For this review, use the dimensioned drawing (mm, ordinates from the lowest corner) and the shaded views. A direction names the side the tool comes from. Coordinates: 2 decimals unless noted, no trailing zeros. Loops run counter-clockwise (first coordinate to the right, second up) from the corner with the lowest first, then second, coordinate; pieces in that order, holes last. Notation, with made-up numbers: M -40,61.25 L -6,61.25 A30 ccw -6,98.25 Z; hole C -7.5,83 d2. An arc over 180 degrees is marked long. Write item = value, one per line. Start each with the question number.
Q1. We need section D-D on x = 15. Give the boundary of the cut face in (y, z), and give its area (3 significant figures).
Q2. For the marked faces 1 and 2, list the 3-axis set-ups (+Z, -Z, +X, -X, +Y, -Y) from which the entire face can be reached by the end or side of a thin tool; tool diameter is ignored.
Q3. Clearance check with flat-ended pins moving along their axes: pin 1 Ø1.5 at (x, z) = (12, 17) entering from +Y; pin 2 Ø10 at (x, y) = (14.5, 12.5) entering from +Z. State where each tip first meets the part, or that it passes through.
Q4. We need section B-B on x = 9. Give the boundary of the cut face in (y, z).
Q5. Mouldability with a two-part tool opening along Y and no side actions: class the marked faces 3, 4 and 5 as released by +Y, released by -Y, zero draft, split by the parting line, or undercut.
Q6. We need section A-A on z = 10. Give the boundary of the cut face in (x, y), and give its area (3 significant figures).
Q7. Wall thickness on probe 1 along X at (y, z) = (1.15, 10); probe 2 along Y at (x, z) = (9, 2.05): over which ranges is each line inside the solid? List them lowest first.
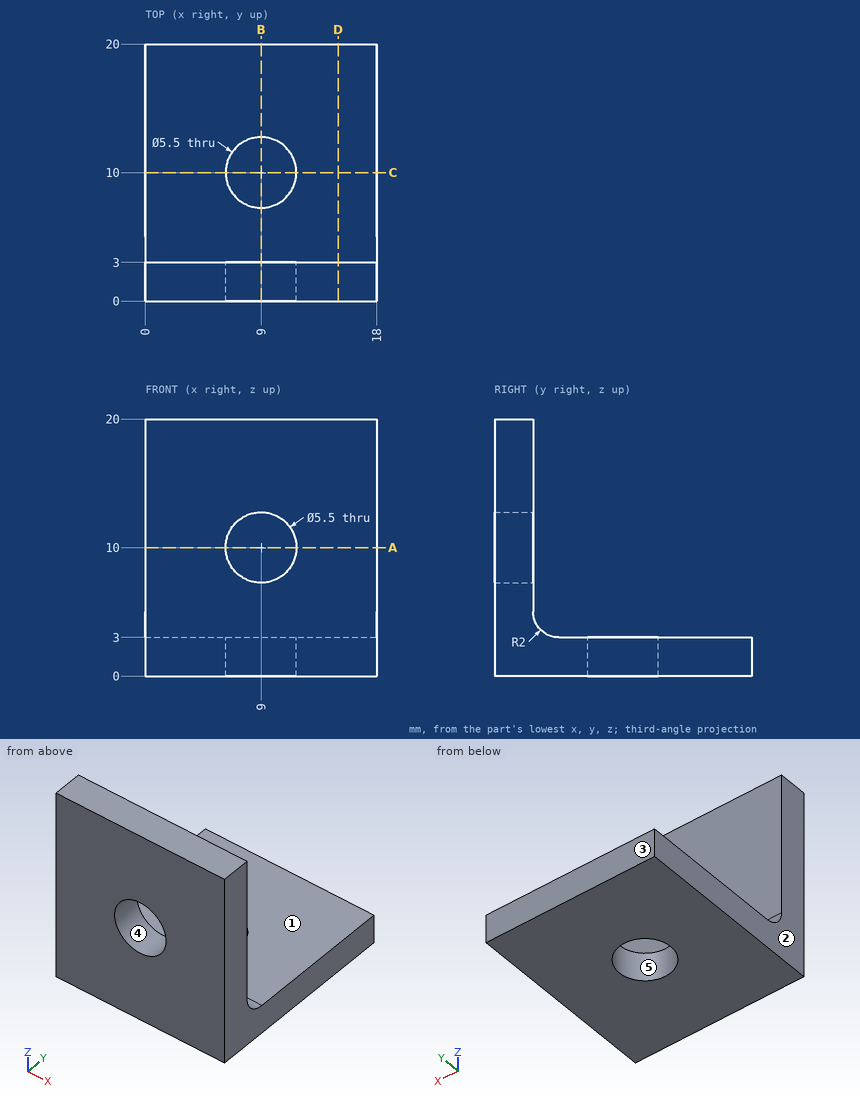
Returned:
q1.outline = M 0,0 L 20,0 L 20,3 L 5,3 A2 cw 3,5 L 3,20 L 0,20 Z
q1.area = 112 mm^2
q2.face_1 = +Z, +X, -X, +Y
q2.face_2 = +Z, -Z, -X, +Y, -Y
q3.pin_1 = 3
q3.pin_2 = 3
q4.outline = M 0,0 L 7.25,0 L 7.25,3 L 5,3 A2 cw 3,5 L 3,7.25 L 0,7.25 Z; M 0,12.75 L 3,12.75 L 3,20 L 0,20 Z; M 12.75,0 L 20,0 L 20,3 L 12.75,3 Z
q5.face_3 = released by +Y
q5.face_4 = zero draft
q5.face_5 = undercut
q6.outline = M 0,0 L 6.25,0 L 6.25,3 L 0,3 Z; M 11.75,0 L 18,0 L 18,3 L 11.75,3 Z
q6.area = 37.5 mm^2
q7.probe_1 = 0 to 6.25, 11.75 to 18
q7.probe_2 = 0 to 7.25, 12.75 to 20
